Check sheet for the modelled part. Datum: model origin and axes. Units: mm. A direction names the side the tool comes from. Round coordinates to 2 decimals unless told otherwise and drop trailing zeros. Order: outer loops, then holes, each group sorted by start corner. A loop starts at its lowest first (then second) coordinate and runs counter-clockwise, first axis right, second up.
Q1. Scan lines: probe 1 along Z at (x, y) = (10, 3); probe 2 along Z at (x, y) = (10, -45.25); probe 3 along Y at (x, z) = (124, 6.5). Record each from-to range of solid material in increasing order.
Q2. Depth check by flat-ended pin: P1, Ø1, axis at y = -59, z = 9, coming from the +X side; P2, Ø11, axis at x = 10, z = 10, coming from the +Y side; P3, Ø9, axis at x = 10, z = 10, coming from the -Y side. Enter the tip coordinate at first touch or a pass-through.
Q3. Cross-section at C-C on x = 127.5. Record the cut outline in (y, z), then the cut area to 3 significant figures.
Q4. Set-up check for faces 4 (the cylindrical face through (106.31, -106.414, 17.895)), 5 (the cylindrical face through (32.59, -95.985, 1.996)), 6 (the cylindrical face through (22, -35.5, 17.9)), 7 (the flat face through (12.3, -5, 12.1)): record each of +Z, -Z, +X, -X, +Y, -Y from which the full face is reachable in a straight line by a thin tool's end or side.
Q5. Cross-section at B-B on y = -66. Record the cut outline in (x, z).
Q6. Mould release check, pull along Z, two halves, no side actions. Record for faces 1 (the cylindrical face through (166.46, -96.52, 2)), 2 (the flat face through (16, 6, 12)), 3 (the cylindrical face through (16, -68, 10)): +Z half, -Z half, draft (parallel to the pull), parting line (faces both ways), or undercut.
Q7. Cross-section at A-A on x = 10. Record the cut outline in (y, z).
from build123d import *

# Parameters (mm, degrees)
F1_DEPTH      = 20
F2_W          = 9
F2_H          = 1
F3_DEPTH      = 20
F4_SIZE       = 0.99999
F6_DEPTH      = 20
F9_DEPTH      = 3
F10_SIZE      = 20
F11_DEPTH     = 6
F13_R         = 2.8
F14_DEPTH     = 130.4192752567
F15_R         = 6
F16_DEPTH     = 76.1192752567
F17_R         = 6
F18_DEPTH     = 6
F19_R         = 15
F20_T1_DEPTH  = 113.7867965644
F20_T3_DEPTH  = 40
F20_T5_DEPTH  = 15.8578643763
F20_T7_DEPTH  = 101.7050718211
F20_T10_ANGLE = 45
F20_T12_ANGLE = 45
F20_T14_ANGLE = 45
F20_T16_ANGLE = 45
F21_SIZE      = 1.5
F22_R         = 20
F23_SIZE      = 2.5


# Not quite as in the source:
# - a fillet or chamfer that OpenCascade refuses, or shapes differently, is made with other operations: its cross-section is extruded or revolved along the edge and cut away or added
# - a fillet or chamfer is up to 0.001 mm smaller than in the source, because OpenCascade refuses the exact size


with BuildPart() as f1:
    # F0 (on Top) → F1 (new body)
    with BuildSketch(Plane.XY):
        Polygon((24, 0), (0, 0), (0, -4), (20, -4), (20, -44.3), (0, -44.3), (0, -48.3), (24, -48.3), align=None)
    extrude(amount=F1_DEPTH)

    # F2 (on face) → F3 (join, through all)
    with BuildSketch(Plane.XY.offset(20)):
        with Locations((10, -4.5)):
            Rectangle(F2_W, F2_H)
        with Locations((10, -43.8)):
            Rectangle(F2_W, F2_H)
    extrude(amount=-F3_DEPTH)

    # F4 (size 1 in the source; OpenCascade refuses exactly that, so slightly less here)
    f4_edges = [f1.edges().sort_by_distance(p)[0] for p in [
        (5.5, -5, 10),
        (14.5, -5, 10),
        (10, -5, 20),
        (10, -5, 0),
        (14.5, -43.3, 10),
        (5.5, -43.3, 10),
        (10, -43.3, 20),
        (10, -43.3, 0),
    ]]
    chamfer(f4_edges, length=F4_SIZE)

    # F5 (on face) → F6 (join, through all)
    with BuildSketch(Plane.XY.offset(20)):
        Polygon((24, -48.3), (0, -48.3), (24, -124.4182752567), (169, -124.4182752567), (169, -94.4182752567), (164, -94.4182752567), (164, -104.4182752567), (24, -104.4182752567), align=None)
    extrude(amount=-F6_DEPTH)

    # F8 (on offset) → F9 (join, symmetric)
    with BuildSketch(Plane.XY.offset(10)):
        Polygon((54, -104.4182752567), (24, 0), (24, -104.4182752567), align=None)
    extrude(amount=F9_DEPTH, both=True)

    # F10
    f10_edges = [f1.edges().sort_by_distance(p)[0] for p in [
        (24, -104.418275, 16.5),
        (24, -104.418275, 3.5),
    ]]
    chamfer(f10_edges, length=F10_SIZE)

    # F11 (add): a face of the model
    f11_faces = [f1.faces().sort_by_distance(p)[0] for p in [
        (12, 0, 10),
    ]]
    extrude(f11_faces, amount=F11_DEPTH)

    # F13 (on face) → F14 (cut, through all)
    with BuildSketch(Plane(origin=(0, 6, 0), x_dir=(-1, 0, 0), z_dir=(0, 1, 0))):
        with Locations((-10, 10)):
            Circle(F13_R)
    extrude(amount=-F14_DEPTH, mode=Mode.SUBTRACT)

    # F15 (on offset) → F16 (cut, through all)
    with BuildSketch(Plane(origin=(0, -48.3, 0), x_dir=(-1, 0, 0), z_dir=(0, 1, 0))):
        with Locations((-10, 10)):
            Circle(F15_R)
    extrude(amount=-F16_DEPTH, mode=Mode.SUBTRACT)

    # F17 (on face) → F18 (cut)
    with BuildSketch(Plane(origin=(0, 6, 0), x_dir=(-1, 0, 0), z_dir=(0, 1, 0))):
        with Locations((-10, 10)):
            Circle(F17_R)
    extrude(amount=-F18_DEPTH, mode=Mode.SUBTRACT)

    # F19
    f19_edges = [f1.edges().sort_by_distance(p)[0] for p in [
        (44, -104.418275, 3.5),
        (24, -84.418275, 3.5),
        (24, -84.418275, 16.5),
        (44, -104.418275, 16.5),
    ]]
    fillet(f19_edges, radius=F19_R)

    # F20: fillet of radius 7 on 12 edges, made by hand

    # F20_s2 → F20_t1 (cut)
    with BuildSketch(Plane.YZ.offset(50.2132034356)):
        with BuildLine():
            ThreePointArc((-104.4182752567, 13), (-106.4685277884, 17.9497474683), (-111.4182752567, 20))
            Line((-111.4182752567, 20), (-104.4182752567, 20))
            Line((-104.4182752567, 20), (-104.4182752567, 13))
        make_face()
        with BuildLine():
            ThreePointArc((-111.4182752567, 0), (-106.4685277884, 2.0502525317), (-104.4182752567, 7))
            Line((-104.4182752567, 7), (-104.4182752567, 0))
            Line((-104.4182752567, 0), (-111.4182752567, 0))
        make_face()
    extrude(amount=F20_T1_DEPTH, mode=Mode.SUBTRACT)

    # F20_s4 → F20_t3 (cut)
    with BuildSketch(Plane.YZ.offset(146.5)):
        with BuildLine():
            ThreePointArc((-101.4182752567, 0), (-96.4685277884, 2.0502525317), (-94.4182752567, 7))
            Line((-94.4182752567, 7), (-94.4182752567, 0))
            Line((-94.4182752567, 0), (-101.4182752567, 0))
        make_face()
        with BuildLine():
            ThreePointArc((-94.4182752567, 13), (-96.4685277884, 17.9497474683), (-101.4182752567, 20))
            Line((-101.4182752567, 20), (-94.4182752567, 20))
            Line((-94.4182752567, 20), (-94.4182752567, 13))
        make_face()
    extrude(amount=F20_T3_DEPTH, mode=Mode.SUBTRACT)

    # F20_s6 → F20_t5 (cut)
    with BuildSketch(Plane(origin=(69.8157393462, -69.8157393462, 0), x_dir=(0, 0, 1), z_dir=(-0.7071067812, 0.7071067812, 0))):
        with BuildLine():
            ThreePointArc((0, -49.7221721416), (2.0502525317, -44.7724246733), (7, -42.7221721416))
            Line((7, -42.7221721416), (0, -42.7221721416))
            Line((0, -42.7221721416), (0, -49.7221721416))
        make_face()
        with BuildLine():
            ThreePointArc((20, -49.7221721416), (17.9497474683, -44.7724246733), (13, -42.7221721416))
            Line((13, -42.7221721416), (20, -42.7221721416))
            Line((20, -42.7221721416), (20, -49.7221721416))
        make_face()
    extrude(amount=F20_T5_DEPTH, mode=Mode.SUBTRACT)

    # F20_s8 → F20_t7 (cut)
    with BuildSketch(Plane.XZ.offset(-23.5)):
        with BuildLine():
            ThreePointArc((17, 0), (21.9497474683, 2.0502525317), (24, 7))
            Line((24, 7), (24, 0))
            Line((24, 0), (17, 0))
        make_face()
        with BuildLine():
            ThreePointArc((24, 13), (21.9497474683, 17.9497474683), (17, 20))
            Line((17, 20), (24, 20))
            Line((24, 20), (24, 13))
        make_face()
    extrude(amount=F20_T7_DEPTH, mode=Mode.SUBTRACT)

    # F20_s9 → F20_t10 (revolve, cut)
    with BuildSketch(Plane.YZ.offset(50.2132034356)):
        with BuildLine():
            ThreePointArc((-111.4182752567, 0), (-106.4685277884, 2.0502525317), (-104.4182752567, 7))
            Line((-104.4182752567, 7), (-104.4182752567, 0))
            Line((-104.4182752567, 0), (-111.4182752567, 0))
        make_face()
    revolve(axis=Axis((50.2132034356, -89.4182752567, 0), (0, 0, -1)), revolution_arc=F20_T10_ANGLE, mode=Mode.SUBTRACT)

    # F20_s11 → F20_t12 (revolve, cut)
    with BuildSketch(Plane(origin=(58.6025359106, -58.6025359106, 0), x_dir=(0, 0, 1), z_dir=(0.7071067812, -0.7071067812, 0))):
        with BuildLine():
            ThreePointArc((0, 49.7221721416), (2.0502525317, 44.7724246733), (7, 42.7221721416))
            Line((7, 42.7221721416), (0, 42.7221721416))
            Line((0, 42.7221721416), (0, 49.7221721416))
        make_face()
    revolve(axis=Axis((39, -78.2050718211, 0), (0, 0, -1)), revolution_arc=F20_T12_ANGLE, mode=Mode.SUBTRACT)

    # F20_s13 → F20_t14 (revolve, cut)
    with BuildSketch(Plane.YZ.offset(50.2132034356)):
        with BuildLine():
            ThreePointArc((-111.4182752567, 20), (-106.4685277884, 17.9497474683), (-104.4182752567, 13))
            Line((-104.4182752567, 13), (-104.4182752567, 20))
            Line((-104.4182752567, 20), (-111.4182752567, 20))
        make_face()
    revolve(axis=Axis((50.2132034356, -89.4182752567, 20), (0, 0, -1)), revolution_arc=F20_T14_ANGLE, mode=Mode.SUBTRACT)

    # F20_s15 → F20_t16 (revolve, cut)
    with BuildSketch(Plane.XZ.offset(78.2050718211)):
        with BuildLine():
            ThreePointArc((17, 20), (21.9497474683, 17.9497474683), (24, 13))
            Line((24, 13), (24, 20))
            Line((24, 20), (17, 20))
        make_face()
    revolve(axis=Axis((39, -78.2050718211, 20), (0, 0, 1)), revolution_arc=F20_T16_ANGLE, mode=Mode.SUBTRACT)

    # F21
    f21_edges = [f1.edges().sort_by_distance(p)[0] for p in [
        (39, -52.209138, 13),
        (39, -52.209138, 7),
    ]]
    chamfer(f21_edges, length=F21_SIZE)

    # F22
    f22_edges = [f1.edges().sort_by_distance(p)[0] for p in [
        (24, -124.418275, 10),
        (169, -124.418275, 10),
    ]]
    fillet(f22_edges, radius=F22_R)

    # F23
    f23_edges = [f1.edges().sort_by_distance(p)[0] for p in [
        (0, 6, 10),
    ]]
    chamfer(f23_edges, length=F23_SIZE)


solid = f1.part
Results found:
1. probe 1: z = 0 to 4, 16 to 20
1. probe 2: z = 0 to 7.2, 12.8 to 20
1. probe 3: y = -124.42 to -104.44
2. P1: stops at x = 41.09
2. P2: stops at y = 0
2. P3: stops at y = -48.3
3. outline: (-124.42, 0) - (-111.42, 0) arc R7 ccw to (-104.42, 7) - (-104.42, 13) arc R7 ccw to (-111.42, 20) - (-124.42, 20) - close
3. area: 379 mm2
4. face 4: +Z, +Y
4. face 5: -Z, +Y
4. face 6: +Z, +X, +Y
4. face 7: +Z, -Z, -X
5. outline: (5.58, 0) - (17, 0) arc R7 ccw to (24, 7) - (41.4, 7) - (42.96, 8.5) - (42.96, 11.5) - (41.4, 13) - (24, 13) arc R7 ccw to (17, 20) - (5.58, 20) - (5.58, 14.06) arc R6 cw (long way) to (5.58, 5.94) - close
6. face 1: -Z half
6. face 2: draft
6. face 3: undercut
7. outline: (-80.02, 0) - (-44.3, 0) - (-43.3, 1) - (-43.3, 7.2) - (-48.3, 7.2) - (-48.3, 4) - (-80.02, 4) - close; (-80.02, 16) - (-48.3, 16) - (-48.3, 12.8) - (-43.3, 12.8) - (-43.3, 19) - (-44.3, 20) - (-80.02, 20) - close; (-5, 1) - (-4, 0) - (6, 0) - (6, 4) - (0, 4) - (0, 7.2) - (-5, 7.2) - close; (-5, 12.8) - (0, 12.8) - (0, 16) - (6, 16) - (6, 20) - (-4, 20) - (-5, 19) - close
